Source: CAD feature listing. Evaluate the final solid. Frame: model axes, mm. A direction names the side the tool comes from. Give positions to 0.01 mm unless a question says otherwise; leave off trailing zeros. Put each result on its own line as item: value.
```python
from build123d import *

# Parameters (mm, degrees)
SKETCH2_W           = 7.9
SKETCH2_H           = 7.9
BOSS_EXTRUDE1_DEPTH = 3.2
SKETCH3_W           = 7.9
SKETCH3_H           = 7.9
BOSS_EXTRUDE2_DEPTH = 3.2
SKETCH7_W           = 7.9
SKETCH7_H           = 3.2
BOSS_EXTRUDE5_DEPTH = 7.2
CUT_EXTRUDE2_DEPTH  = 8.2


with BuildPart() as part:
    # Sketch2 → Boss-Extrude1 (new body)
    with BuildSketch(Plane(origin=(0, 0, 0), x_dir=(1, 0, 0), z_dir=(0, 1, 0))):
        with Locations((3.95, 3.95)):
            Rectangle(SKETCH2_W, SKETCH2_H)
    extrude(amount=BOSS_EXTRUDE1_DEPTH)



with BuildPart() as body_2:
    # Sketch3 → Boss-Extrude2 (new body)
    with BuildSketch(Plane(origin=(0, 3.2, 0), x_dir=(1, 0, 0), z_dir=(0, 1, 0))):
        with Locations((11.85, 3.95)):
            Rectangle(SKETCH3_W, SKETCH3_H)
    extrude(amount=BOSS_EXTRUDE2_DEPTH)


with BuildPart() as part_1:
    add(part.part)

    add(body_2.part)  # Boss-Extrude5 merges body 2
    # Sketch7 → Boss-Extrude5 (add)
    with BuildSketch(Plane.ZY.offset(-7.9)):
        with Locations((-3.95, 4.8)):
            Rectangle(SKETCH7_W, SKETCH7_H)
    extrude(amount=BOSS_EXTRUDE5_DEPTH)

    # Sketch4 → Cut-Extrude2 (cut)
    with BuildSketch(Plane(origin=(0, 0, -7.9), x_dir=(-1, 0, 0), z_dir=(0, 0, -1))):
        with BuildLine():
            Line((-15.8, 6.4), (0, 6.4))
            Line((0, 6.4), (0, 0))
            add(Edge.make_bspline(
                [(-15.8, 6.4), (-6.684647753, 6.042665729), (0, 0)],
                knots=[0, 0, 0, 1, 1, 1], degree=2))
        make_face()
    extrude(amount=-CUT_EXTRUDE2_DEPTH, mode=Mode.SUBTRACT)


solid = part_1.part
```
(1) Reachability of faces 1 (the flat face through (15.8, 5, -4)), 2 (the flat face through (7.9, 2, -4)) from +Z, -Z, +X, -X, +Y, -Y: full face, straight path, thin tool, end or side. Return the list, or none.
Calculated:
face 1: +Z, -Z, +X, +Y, -Y
face 2: +Z, -Z, +X, -Y
(2) First-contact query: P1, Ø2.5, axis at x = 12, z = -3.5, coming from the -Y side; P2, Ø3, axis at x = 11, z = -6.5, coming from the +Y side; P3, Ø3.5, axis at y = 1, z = -2.5, coming from the +X side. Flat tips, straight axial feed; report the tip coordinate or a pass-through.
Calculated:
P1: stops at y = 3.2
P2: stops at y = 6.07
P3: stops at x = 7.9
(3) Line query: probe 1 along X at (y, z) = (1, -3.5); probe 2 along Y at (x, z) = (3.5, -4.75); probe 3 along Y at (x, z) = (6.5, -1.5). Output: solid intervals per line, ascending. Write a range as from..to.
Calculated:
probe 1: x = 1.17..7.9
probe 2: y = 0..2.67
probe 3: y = 0..4.28
